Autodesk Fusion 360 part; units mm, degrees
sketch "Sketch1" plane through (0, 0, 0) normal (0, 0, 1) x (1, 0, 0)
  line L0 (33.0292, 88.6269) -> (55.0292, 88.6269)
  line L1 (33.0292, 40.6269) -> (55.0292, 40.6269)
  arc A0 (33.0292, 88.6269) -> (33.0292, 40.6269) centre (40.0292, 64.6269) ccw
  arc A1 (55.0292, 40.6269) -> (55.0292, 88.6269) centre (48.0292, 64.6269) ccw
  arc A2 (55.3093, 38.6269) -> (55.3093, 90.6269) centre (48.0292, 64.6269) ccw
  line L2 (32.7491, 38.6269) -> (55.3093, 38.6269)
  line L3 (32.7491, 90.6269) -> (55.3093, 90.6269)
  arc A3 (32.7491, 90.6269) -> (32.7491, 38.6269) centre (40.0292, 64.6269) ccw
  arc A4 (33.0292, 88.6269) -> (33.0292, 40.6269) centre (40.0292, 64.6269) ccw
  arc A5 (26.1098, 102.1269) -> (26.1098, 27.1269) centre (40.0292, 64.6269) ccw
  arc A6 (61.9486, 27.1269) -> (61.9486, 102.1269) centre (48.0292, 64.6269) ccw
  line L4 (26.1098, 102.1269) -> (61.9486, 102.1269)
  line L5 (26.1098, 27.1269) -> (61.9486, 27.1269)
  point P0 (15.0292, 64.6269)
  point P1 (73.0292, 64.6269)
  point P2 (75.0292, 64.6269)
  point P3 (13.0292, 64.6269)
  dimension "d5" = 50
  dimension "d6" = 48
  dimension "d10" = 58
  dimension "d23" = 52
  dimension "d24" = 62
  dimension "d25" = 27
  dimension "d26" = 27
  dimension "d27" = 8
  dimension "d28" = 8
  dimension "d31" = 50
  dimension "d32" = 48
  dimension "d33" = 75
  dimension "d34" = 40
  dimension "d35" = 75
  dimension "d36" = 40
  dimension "d37" = 8
extrude "Extrude1" add sketch "Sketch1" along normal blind 20 contours A2 L2 L3 A3
extrude "Extrude2" add sketch "Sketch1" against normal blind 2 contours A2 L2 L3 A3 | A5 A6 L4 L5
chamfer "Chamfer1" distance 4 angle 45 4 edges at (44.0292, 90.6269, 0) (13.0292, 64.6269, 0) (75.0292, 64.6269, 0) (44.0292, 38.6269, 0)
Input: part model. Units: mm. Frame: model coordinates. A direction names the side the tool comes from. Give positions to 0.01 mm unless a question says otherwise; leave off trailing zeros. Write each loop counter-clockwise with the first axis right and the second up, starting at its lowest first coordinate (ties: lowest second). Pieces come first, ordered by that corner, then holes. Notation, with made-up numbers: (87.25, 43) - (121.25, 43) arc R14 cw to (121.25, 54) - close; hole circle Ø3 at (-21.5, -12). An arc over 180 degrees is marked (long way). Write item = value, one per line. Start each with the question number.
1. Ray query, L1, parallel to Y at x = 53, z = 17.5; L2, parallel to X at y = 64, z = 10.5; L3, parallel to Y at x = 17, z = 1.5. Return the intervals inside material, ascending.
2. First-contact query: pin 1 Ø10 at (x, y) = (41.5, 92.5) entering from +Z; pin 2 Ø8 at (x, z) = (12.5, 15) entering from -Y; pin 3 Ø1.5 at (x, z) = (61.5, 6) entering from -Y; pin 4 Ø12 at (y, z) = (60.5, 13.5) entering from -X. Flat tips, straight axial feed; report the tip coordinate or a pass-through.
3. Section query B-B, the plane z = 10. Output: boundary loops of the cut face in (x, y).
4. Section query A-A, the plane x = 44.5. Output: boundary loops of the cut face in (y, z), then the cut area to 3 significant figures.
5. Access query for faces 1 (the cylindrical face through (75.025, 65.117, 11.888)), 2 (the flat face through (44, 90.627, 12)), 3 (the flat face through (44, 95, 0)), 4 (the cylindrical face through (13.034, 64.136, 11.888)). Directions: +Z, -Z, +X, -X, +Y, -Y. A direction counts if a zero-diameter tool reaches every point of the face in a straight line with its end or side. Return the directions, or none.
6. Mould query, pull axis Y, two halves, no side actions, for faces 5 (the flat face through (44, 102.127, -1)), 6 (the cylindrical face through (15.033, 64.176, 8.846)), 7 (the flat face through (44.195, 36.599, 1.972)). Classes: released by +Y, released by -Y, zero draft, split by the parting line, or undercut.
7. Section query C-C, the plane z = 1. Output: boundary loops of the cut face in (x, y), then the cut area to 3 significant figures.
Check sheet entries:
q1.L1 = 38.63 to 40.63, 88.63 to 90.63
q1.L2 = 13.04 to 15.04, 73.02 to 75.02
q1.L3 = 46.19 to 54.9, 74.36 to 83.06
q2.pin_1 = 20
q2.pin_2 = 51.38
q2.pin_3 = 40.81
q2.pin_4 = 13.03
q3.outline = (32.75, 38.63) - (55.31, 38.63) arc R27 ccw to (55.31, 90.63) - (32.75, 90.63) arc R27 ccw to start; hole (33.03, 40.63) - (55.03, 40.63) arc R25 ccw to (55.03, 88.63) - (33.03, 88.63) arc R25 ccw to start
q4.outline = (27.13, -2) - (40.63, -2) - (40.63, 20) - (38.63, 20) - (38.63, 4) - (34.63, 0) - (27.13, 0) - close; (88.63, -2) - (102.13, -2) - (102.13, 0) - (94.63, 0) - (90.63, 4) - (90.63, 20) - (88.63, 20) - close
q4.area = 150 mm2
q5.face_1 = +Z, +X
q5.face_2 = +Z, +X, -X, +Y
q5.face_3 = +Z
q5.face_4 = +Z, -X
q6.face_5 = released by +Y
q6.face_6 = undercut
q6.face_7 = released by -Y
q7.outline = (32.35, 35.63) - (55.71, 35.63) arc R30 ccw to (55.71, 93.63) - (32.35, 93.63) arc R30 ccw to start; hole (33.03, 40.63) - (55.03, 40.63) arc R25 ccw to (55.03, 88.63) - (33.03, 88.63) arc R25 ccw to start
q7.area = 942 mm2
